Part model, mm, in its own coordinate system. Face numbers are marked on the shaded views. Give positions to 0.01 mm unless a question says otherwise; leave off trailing zeros. Order: outer loops, then holes, each group sorted by start corner. A loop starts at its lowest first (then second) coordinate and runs counter-clockwise, first axis right, second up. Notation, with made-up numbers: M 29.25,88.5 L 64.25,88.5 A26 ccw 64.25,115.5 Z; hole C -37,-25 d1. An arc over 180 degrees is marked long. Return JSON: item names as keys, results as strings.
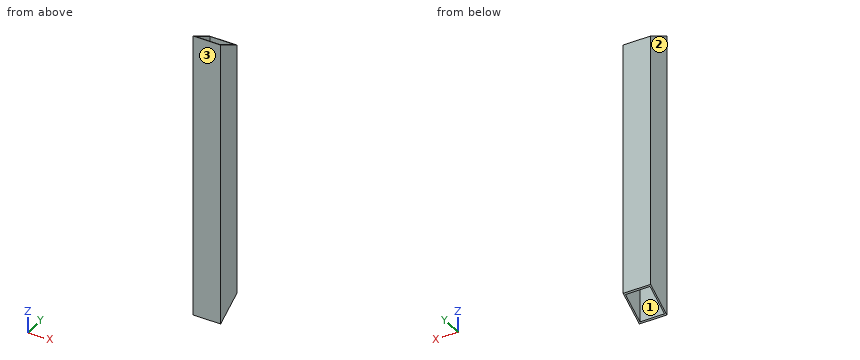
from build123d import *

# Parameters (mm, degrees)
SKETCH1_W               = 19
SKETCH1_H               = 19
SKETCH1_W_2             = 17
SKETCH1_H_2             = 17
BOSS_EXTRUDE1_DEPTH     = 200
CUT_EXTRUDE1_DEPTH      = 1
CUT_EXTRUDE1_DEPTH_BACK = 20
CUT_EXTRUDE2_DEPTH      = 1
CUT_EXTRUDE2_DEPTH_BACK = 20


with BuildPart() as part:
    # Sketch1 → Boss-Extrude1 (new body)
    with BuildSketch(Plane.XY):
        Rectangle(SKETCH1_W, SKETCH1_H)
        Rectangle(SKETCH1_W_2, SKETCH1_H_2, mode=Mode.SUBTRACT)
    extrude(amount=BOSS_EXTRUDE1_DEPTH)

    # Sketch2 → Cut-Extrude1 (cut, two sides)
    with BuildSketch(Plane(origin=(9.5, 0, 0), x_dir=(0, 0, -1), z_dir=(1, 0, 0))) as cut_extrude1_sk:
        Polygon((-405.900472872, -366.130080316), (-200, -9.5), (-189.030344885, 9.5), (16.870127986, 366.130080316), (-696.390032646, 777.931026059), (-1119.160633503, 45.670865427), align=None)
    extrude(amount=CUT_EXTRUDE1_DEPTH, mode=Mode.SUBTRACT)
    extrude(cut_extrude1_sk.sketch, amount=-CUT_EXTRUDE1_DEPTH_BACK, mode=Mode.SUBTRACT)

    # Sketch3 → Cut-Extrude2 (cut, two sides)
    with BuildSketch(Plane(origin=(9.5, 0, 0), x_dir=(0, 0, -1), z_dir=(1, 0, 0))) as cut_extrude2_sk:
        Polygon((205.900472872, -366.130080316), (0, -9.5), (-10.969655115, 9.5), (-216.870127986, 366.130080316), (496.390032646, 777.931026059), (919.160633503, 45.670865427), align=None)
    extrude(amount=CUT_EXTRUDE2_DEPTH, mode=Mode.SUBTRACT)
    extrude(cut_extrude2_sk.sketch, amount=-CUT_EXTRUDE2_DEPTH_BACK, mode=Mode.SUBTRACT)


solid = part.part
Q1. Pin check, flat tips, straight feed: pin 1 (6 mm diameter, centred on x = 7, y = 4.5, fed in from +Z); pin 2 (1.5 mm diameter, centred on x = -4.5, y = 6.5, fed in from +Z). Stop position of each tip, or through.
Established:
{"pin 1": "stops at z = 193.42", "pin 2": "passes through"}
Q2. Two-plate mould, pull along X, no slides. Class the marked faces 1, 2 and 3: +X half, -X half, draft (parallel to the pull), parting line (faces both ways), or undercut.
Established:
{"face 1": "undercut", "face 2": "-X half", "face 3": "draft"}
Q3. Band-saw the part on A-A (x = 6.75). Give the cut face in (y, z), then the cut area to 3 significant figures.
Established:
{"outline": "M -9.5,0 L -8.5,0.58 L -8.5,199.42 L -9.5,200 Z; M 8.5,10.39 L 9.5,10.97 L 9.5,189.03 L 8.5,189.61 Z", "area": "378 mm²"}
Q4. Band-saw the part on C-C (z = 34). Give the cut face in (x, y), then the cut area to 3 significant figures.
Established:
{"outline": "M -9.5,-9.5 L 9.5,-9.5 L 9.5,9.5 L -9.5,9.5 Z; hole M -8.5,-8.5 L 8.5,-8.5 L 8.5,8.5 L -8.5,8.5 Z", "area": "72.0 mm²"}
Q5. Probe line 1 along X through (y, z) = (-3.75, 129); line 2 along Y through (x, z) = (-6.5, 189.5). List the from-to ranges inside material, lowest first.
Established:
{"line 1": "x = -9.5 to -8.5, 8.5 to 9.5", "line 2": "y = -9.5 to -8.5, 8.5 to 8.69"}
Q6. Band-saw the part on B-B (y = 5.5). Give the cut face in (x, z).
Established:
{"outline": "M -9.5,8.66 L -8.5,8.66 L -8.5,191.34 L -9.5,191.34 Z; M 8.5,8.66 L 9.5,8.66 L 9.5,191.34 L 8.5,191.34 Z"}
